Build history of the part. All positions in model axes, mm. A direction names the side the tool comes from. Give positions to 0.01 mm unless a question says otherwise; leave off trailing zeros. Order: outer loops, then holes, each group sorted by start corner. A loop starts at its lowest first (then second) coordinate and runs counter-clockwise, first axis right, second up. Notation, with made-up numbers: (3, 31) -> (45, 31) arc R13 ccw to (45, 52) -> close; hole circle Ø9 at (78.25, 2.5). An arc over 180 degrees is marked (long way). Use a Markdown table: item, result. Add a question column.
```python
from build123d import *

# Parameters (mm, degrees)
F0_R     = 3.175
F1_DEPTH = 7.62
F2_T     = -0.508
F0_R_2   = 6.35
F3_DEPTH = 0.508


with BuildPart() as f1:
    # F0 (on Top) → F1 (new body)
    with BuildSketch(Plane.XY):
        Circle(F0_R)
    extrude(amount=F1_DEPTH)

    # F2
    f2_openings = [f1.faces().sort_by_distance(p)[0] for p in [
        (0, 0, 7.62),
    ]]
    offset(amount=F2_T, openings=f2_openings)

    # F0 (on Top) → F3 (join)
    with BuildSketch(Plane.XY):
        Circle(F0_R_2)
        Circle(F0_R, mode=Mode.SUBTRACT)
    extrude(amount=F3_DEPTH)


solid = f1.part
```
(1) Band-saw the part on C-C on z = 7.25. Give the cut face in (x, y) (3 decimals).
(2) Wall check: probe 1 along Y at (x, z) = (0, 3) (3 decimals); probe 2 along Z at (x, y) = (-5, -1.25); probe 3 along Y at (x, z) = (-1, 2). Give the ranges that are in metal, low to high.
(3) Mould opens along X. For faces 3 (the face through (-1.38, -6.2, 0.25)), 4 (the face through (0, 0, 0)), 5 (the face through (1.231, -2.366, 4.014)) say: released by +X, released by -X, zero draft, split by the parting line, or undercut.
(4) Pin check, flat tips, straight feed: pin 1 Ø1.5 at (x, z) = (1.5, 3) entering from -Y; pin 2 Ø1.5 at (y, z) = (2.5, 2) entering from +X; pin 3 Ø4 at (y, z) = (-3.5, 5) entering from +X. Stop position of each tip, or through.
(5) Band-saw the part on D-D on x = 3. Give the cut face in (y, z).
(6) Tool access for faces 1 (the face through (-2, 2, 7.62)), 2 (the face through (0, 0, 0.508)): list every direction of +Z, -Z, +X, -X, +Y, -Y with a clear straight run to the whole face (end or side of a thin tool).
(7) Band-saw the part on A-A on x = 0. Give the cut face in (y, z) (3 decimals), plus the area to 3 significant figures.
Response:
| question | item | result |
|---|---|---|
| 1 | outline | circle Ø6.35 at (0, 0); hole circle Ø5.334 at (0, 0) |
| 2 | probe 1 | y = -3.175 to -2.667, 2.667 to 3.175 |
| 2 | probe 2 | z = 0 to 0.51 |
| 2 | probe 3 | y = -3.01 to -2.47, 2.47 to 3.01 |
| 3 | face 3 | split by the parting line |
| 3 | face 4 | zero draft |
| 3 | face 5 | undercut |
| 4 | pin 1 | stops at y = -3.09 |
| 4 | pin 2 | stops at x = 2.65 |
| 4 | pin 3 | stops at x = 2.8 |
| 5 | outline | (-5.6, 0) -> (5.6, 0) -> (5.6, 0.51) -> (1.04, 0.51) -> (1.04, 7.62) -> (-1.04, 7.62) -> (-1.04, 0.51) -> (-5.6, 0.51) -> close |
| 6 | face 1 | +Z, +X, -X, +Y, -Y |
| 6 | face 2 | +Z |
| 7 | outline | (-6.35, 0) -> (6.35, 0) -> (6.35, 0.508) -> (3.175, 0.508) -> (3.175, 7.62) -> (2.667, 7.62) -> (2.667, 0.508) -> (-2.667, 0.508) -> (-2.667, 7.62) -> (-3.175, 7.62) -> (-3.175, 0.508) -> (-6.35, 0.508) -> close |
| 7 | area | 13.7 mm² |
